from build123d import *
from build123d.topology import SkipClean

# Parameters (mm, degrees)
SKETCH1_R           = 1.8
BOSS_EXTRUDE1_DEPTH = 4
FILLET1_R           = 4
CUT_EXTRUDE2_REACH  = 103.08
BOSS_EXTRUDE3_START = 5.55799
BOSS_EXTRUDE3_DEPTH = 5.55799
SKETCH6_R           = 1.8
CUT_EXTRUDE3_DEPTH  = 102.153572382
BOSS_EXTRUDE6_START = 0.56
SKETCH17_R          = 6
SKETCH17_R_2        = 1.8
BOSS_EXTRUDE6_DEPTH = 0.56
CUT_EXTRUDE13_START = -2.56
SKETCH18_R          = 6
SKETCH18_R_2        = 1.8
CUT_EXTRUDE13_DEPTH = 2.56
BOSS_EXTRUDE7_START = 4.99799
SKETCH19_R          = 6
SKETCH19_R_2        = 3.25
BOSS_EXTRUDE7_DEPTH = 4.99799
SKETCH20_R          = 6
SKETCH20_R_2        = 3.25
BOSS_EXTRUDE8_DEPTH = 2.56
SKETCH21_W          = 180.141886337
SKETCH21_H          = 87.597084555
CUT_EXTRUDE14_DEPTH = 1


with BuildPart() as part:
    # Sketch1 → Boss-Extrude1 (new body)
    with BuildSketch(Plane(origin=(0, 0, 0), x_dir=(1, 0, 0), z_dir=(0, 1, 0))):
        with BuildLine():
            Line((-61.369632465, 35.431773824), (0, 0))
            Line((0, 0), (61.369632465, 35.431773824))
            ThreePointArc((61.369632465, 35.431773824), (70.968700885, 38.119022954), (64.834981957, 45.97656166))
            Line((64.834981957, 45.97656166), (53.646129321, 71.567722497))
            Line((53.646129321, 71.567722497), (49.879862047, 70.196913315))
            Line((49.879862047, 70.196913315), (54.252017225, 60.196913315))
            Line((54.252017225, 60.196913315), (-54.252017225, 60.196913315))
            Line((-54.252017225, 60.196913315), (-49.879862047, 70.196913315))
            Line((-49.879862047, 70.196913315), (-53.646129321, 71.567722497))
            Line((-53.646129321, 71.567722497), (-64.834981957, 45.97656166))
            ThreePointArc((-64.834981957, 45.97656166), (-70.968700885, 38.119022954), (-61.369632465, 35.431773824))
        make_face()
        with Locations(Location((-65.268611951, 39.992251756, 0), (0, 0, 270))):
            Circle(SKETCH1_R, mode=Mode.SUBTRACT)
        with Locations(Location((65.268611951, 39.992251756, 0), (0, 0, 270))):
            Circle(SKETCH1_R, mode=Mode.SUBTRACT)
    extrude(amount=BOSS_EXTRUDE1_DEPTH)

    # Fillet1
    fillet1_edges = [part.edges().sort_by_distance(p)[0] for p in [
        (-54.252017225, 2, -60.196913315),
        (54.252017225, 2, -60.196913315),
    ]]
    fillet(fillet1_edges, radius=FILLET1_R)

    # Sketch4 → Cut-Extrude2 (cut, up to next)
    with BuildSketch(Plane(origin=(0, 4, 0), x_dir=(1, 0, 0), z_dir=(0, 1, 0)), mode=Mode.PRIVATE) as cut_extrude2_sk1:
        Polygon((6, 13.464101615), (43.301270189, 35), (40.301270189, 40.196152423), (6, 20.392304845), align=None)
    cut_extrude2_tool1 = extrude(cut_extrude2_sk1.sketch, amount=-CUT_EXTRUDE2_REACH, mode=Mode.PRIVATE) & part.part
    # Sketch4 → Cut-Extrude2 (cut, up to next)
    with BuildSketch(Plane(origin=(0, 4, 0), x_dir=(1, 0, 0), z_dir=(0, 1, 0)), mode=Mode.PRIVATE) as cut_extrude2_sk2:
        Polygon((-43.301270189, 35), (-6, 13.464101615), (-6, 20.392304845), (-40.301270189, 40.196152423), align=None)
    cut_extrude2_tool2 = extrude(cut_extrude2_sk2.sketch, amount=-CUT_EXTRUDE2_REACH, mode=Mode.PRIVATE) & part.part
    add(cut_extrude2_tool1.solids().sort_by_distance((23.91111, 4, -27.220808))[0], mode=Mode.SUBTRACT)
    add(cut_extrude2_tool2.solids().sort_by_distance((-23.91111, 4, -27.220808))[0], mode=Mode.SUBTRACT)

    # Sketch5 → Boss-Extrude3 (add)
    with BuildSketch(Plane.XZ.offset(BOSS_EXTRUDE3_START)):
        with BuildLine():
            Line((-64.834981957, -45.97656166), (-53.646129321, -71.567722497))
            Line((-53.646129321, -71.567722497), (-49.879862047, -70.196913315))
            Line((-49.879862047, -70.196913315), (-51.802560936, -65.79931348))
            Line((-51.802560936, -65.79931348), (-61.169969855, -44.374161496))
            ThreePointArc((-61.169969855, -44.374161496), (-62.865011704, -45.48976991), (-64.834981957, -45.97656166))
        make_face()
        with BuildLine():
            ThreePointArc((-61.369632465, -35.431773824), (-60.072459528, -36.992251756), (-59.369632465, -38.895875439))
            Line((-59.369632465, -38.895875439), (0, -4.618802154))
            Line((0, -4.618802154), (59.369632465, -38.895875439))
            ThreePointArc((59.369632465, -38.895875439), (60.072459528, -36.992251756), (61.369632465, -35.431773824))
            Line((61.369632465, -35.431773824), (0, 0))
            Line((0, 0), (-61.369632465, -35.431773824))
        make_face()
        with BuildLine():
            ThreePointArc((64.834981957, -45.97656166), (62.865011704, -45.48976991), (61.169969855, -44.374161496))
            Line((61.169969855, -44.374161496), (51.802560936, -65.79931348))
            Line((51.802560936, -65.79931348), (49.879862047, -70.196913315))
            Line((49.879862047, -70.196913315), (53.646129321, -71.567722497))
            Line((53.646129321, -71.567722497), (64.834981957, -45.97656166))
        make_face()
    extrude(amount=-BOSS_EXTRUDE3_DEPTH)

    # Sketch6 → Cut-Extrude3 (cut, through all)
    with BuildSketch(Plane.XZ):
        with Locations(Location((-21.3, -52.196913315, 0), (0, 0, 270))):
            Circle(SKETCH6_R)
        with Locations(Location((21.3, -52.196913315, 0), (0, 0, 270))):
            Circle(SKETCH6_R)
    extrude(amount=-CUT_EXTRUDE3_DEPTH, mode=Mode.SUBTRACT)

    # Sketch17 → Boss-Extrude6 (add)
    # profile 1 of 2: a face of its own
    with BuildSketch(Plane.XZ.offset(BOSS_EXTRUDE6_START)):
        with Locations((65.268611951, -39.992251756)):
            Circle(SKETCH17_R)
        with Locations(Location((65.268611951, -39.992251756, 0), (0, 0, 270))):
            Circle(SKETCH17_R_2, mode=Mode.SUBTRACT)
    # profile 2 of 2: a face of its own
    with BuildSketch(Plane.XZ.offset(BOSS_EXTRUDE6_START)):
        with Locations((-65.268611951, -39.992251756)):
            Circle(SKETCH17_R)
        with Locations(Location((-65.268611951, -39.992251756, 0), (0, 0, 270))):
            Circle(SKETCH17_R_2, mode=Mode.SUBTRACT)
    extrude(amount=-BOSS_EXTRUDE6_DEPTH)

    # Sketch18 → Cut-Extrude13 (cut)
    # profile 1 of 2: a face of its own
    with BuildSketch(Plane(origin=(0, 4, 0), x_dir=(1, 0, 0), z_dir=(0, 1, 0)).offset(CUT_EXTRUDE13_START)):
        with Locations((-65.268611951, 39.992251756)):
            Circle(SKETCH18_R)
        with Locations(Location((-65.268611951, 39.992251756, 0), (0, 0, 90))):
            Circle(SKETCH18_R_2, mode=Mode.SUBTRACT)
    # profile 2 of 2: a face of its own
    with BuildSketch(Plane(origin=(0, 4, 0), x_dir=(1, 0, 0), z_dir=(0, 1, 0)).offset(CUT_EXTRUDE13_START)):
        with Locations((65.268611951, 39.992251756)):
            Circle(SKETCH18_R)
        with Locations(Location((65.268611951, 39.992251756, 0), (0, 0, 90))):
            Circle(SKETCH18_R_2, mode=Mode.SUBTRACT)
    extrude(amount=CUT_EXTRUDE13_DEPTH, mode=Mode.SUBTRACT)

    # Sketch19 → Boss-Extrude7 (add)
    # profile 1 of 2: a face of its own
    with BuildSketch(Plane.XZ.offset(0.56).offset(BOSS_EXTRUDE7_START)):
        with Locations((-65.268611951, -39.992251756)):
            Circle(SKETCH19_R)
        with Locations(Location((-65.268611951, -39.992251756, 0), (0, 0, 270))):
            Circle(SKETCH19_R_2, mode=Mode.SUBTRACT)
    # profile 2 of 2: a face of its own
    with BuildSketch(Plane.XZ.offset(0.56).offset(BOSS_EXTRUDE7_START)):
        with Locations((65.268611951, -39.992251756)):
            Circle(SKETCH19_R)
        with Locations(Location((65.268611951, -39.992251756, 0), (0, 0, 270))):
            Circle(SKETCH19_R_2, mode=Mode.SUBTRACT)
    extrude(amount=-BOSS_EXTRUDE7_DEPTH)

    # Sketch20 → Boss-Extrude8 (add)
    # profile 1 of 2: a face of its own
    with BuildSketch(Plane(origin=(0, 1.44, 0), x_dir=(1, 0, 0), z_dir=(0, 1, 0))):
        with Locations((-65.268611951, 39.992251756)):
            Circle(SKETCH20_R)
        with Locations(Location((-65.268611951, 39.992251756, 0), (0, 0, 90))):
            Circle(SKETCH20_R_2, mode=Mode.SUBTRACT)
    # profile 2 of 2: a face of its own
    with BuildSketch(Plane(origin=(0, 1.44, 0), x_dir=(1, 0, 0), z_dir=(0, 1, 0))):
        with Locations((65.268611951, 39.992251756)):
            Circle(SKETCH20_R)
        with Locations(Location((65.268611951, 39.992251756, 0), (0, 0, 90))):
            Circle(SKETCH20_R_2, mode=Mode.SUBTRACT)
    extrude(amount=BOSS_EXTRUDE8_DEPTH)

    # Sketch21 → Cut-Extrude14 (cut)
    with SkipClean():  # the faces are left unmerged after this step: merging them gives an invalid solid
        with BuildSketch(Plane(origin=(0, 4, 0), x_dir=(1, 0, 0), z_dir=(0, 1, 0))):
            with Locations((-2.136514257, 36.289877784)):
                Rectangle(SKETCH21_W, SKETCH21_H)
        extrude(amount=-CUT_EXTRUDE14_DEPTH, mode=Mode.SUBTRACT)


solid = part.part
CAD build for the part. Positions are in the model's coordinates, mm. A direction names the side the tool comes from. Round coordinates to 2 decimals unless told otherwise and drop trailing zeros. Loops run counter-clockwise (first coordinate to the right, second up) from the corner with the lowest first, then second, coordinate; pieces in that order, holes last.
(1) Cut at A-A (x = -13). Give the cut face in (y, z).
(2) Cut at B-B (z = -28). Give the cut face in (x, y), plus the area to 3 significant figures.
(3) Two-plate mould, pull along Z, no slides. Class faces 4 (the cylindrical face through (-71.02, -1.34, -38.28)), 5 (the flat face through (-1, 3, -36)), 6 (the cylindrical face through (51.454, 1.521, -61.961)), 7 (the cylindrical face through (-19.515, 1.479, -51.963)): +Z half, -Z half, draft (parallel to the pull), parting line (faces both ways), or undercut.
(4) Cut at C-C (y = -4). Give the cut face in (x, z).
(5) Drop flat-ended pins along their axis: pin 1 (2.5 mm diameter, centred on x = -14.5, y = 1, fed in from -Z); pin 2 (3 mm diameter, centred on x = -21.3, z = -52.2, fed in from +Y); pin 3 (2 mm diameter, centred on x = 14, y = -4.5, fed in from +Z); pin 4 (5 mm diameter, centred on x = -65.27, z = -39.99, fed in from -Y). Give the stop position or say it passes through.
(6) Wall check: line 1 along X through (y, z) = (-0.25, -35); line 2 along X through (y, z) = (0.75, -30); line 3 along X through (y, z) = (-1.5, -41.5). Give the ranges that are in metal, low to high.
(7) Which spindle directions (+Z, -Z, +X, -X, +Y, -Y) get a long thin tool onto all of the face, cutting with end or side? Do faces 1 (the flat face through (-1, 0, -42)), 2 (the flat face through (-63.9, 1.44, -38.6)), 3 (the flat face through (24.39, 1.52, -24.08)). Say none if no direction does.
(8) Cut at D-D (x = 21.3). Give the cut face in (y, z).
Findings below:
1. outline: (-5.56, -12.12) - (0, -12.12) - (0, -17.51) - (3, -17.51) - (3, -7.51) - (-5.56, -7.51) - close; (0, -60.2) - (3, -60.2) - (3, -24.43) - (0, -24.43) - close
2. outline: (-48.5, -5.56) - (-40.5, -5.56) - (-40.5, 0) - (-31.18, 0) - (-31.18, 3) - (-48.5, 3) - close; (-19.18, 0) - (19.18, 0) - (19.18, 3) - (-19.18, 3) - close; (31.18, 0) - (40.5, 0) - (40.5, -5.56) - (48.5, -5.56) - (48.5, 3) - (31.18, 3) - close
2. area: 308 mm2
3. face 4: parting line
3. face 5: draft
3. face 6: undercut
3. face 7: undercut
4. outline: (-64.83, -45.98) - (-53.65, -71.57) - (-49.88, -70.2) - (-61.17, -44.37) arc R6 ccw to (-59.37, -38.9) - (0, -4.62) - (59.37, -38.9) arc R6 ccw to (61.17, -44.37) - (49.88, -70.2) - (53.65, -71.57) - (64.83, -45.98) arc R6 ccw (long way) to (61.37, -35.43) - (0, 0) - (-61.37, -35.43) arc R6 ccw (long way) to start; hole circle Ø6.5 at (-65.27, -39.99); hole circle Ø6.5 at (65.27, -39.99)
5. pin 1: stops at z = -60.2
5. pin 2: passes through
5. pin 3: stops at z = -7.51
5. pin 4: stops at y = -0.56
6. line 1: x = -68.6 to -61.94, -60.62 to -52.62, 52.62 to 60.62, 61.94 to 68.6
6. line 2: x = -51.96 to -34.64, -22.64 to 22.64, 34.64 to 51.96
6. line 3: x = -71.08 to -68.15, -62.39 to -59.46, 59.46 to 62.39, 68.15 to 71.08
7. face 1: -Y
7. face 2: +Y
7. face 3: +Y, -Y
8. outline: (-5.56, -16.92) - (0, -16.92) - (0, -22.3) - (3, -22.3) - (3, -12.3) - (-5.56, -12.3) - close; (0, -60.2) - (3, -60.2) - (3, -54) - (0, -54) - close; (0, -50.4) - (3, -50.4) - (3, -29.23) - (0, -29.23) - close
